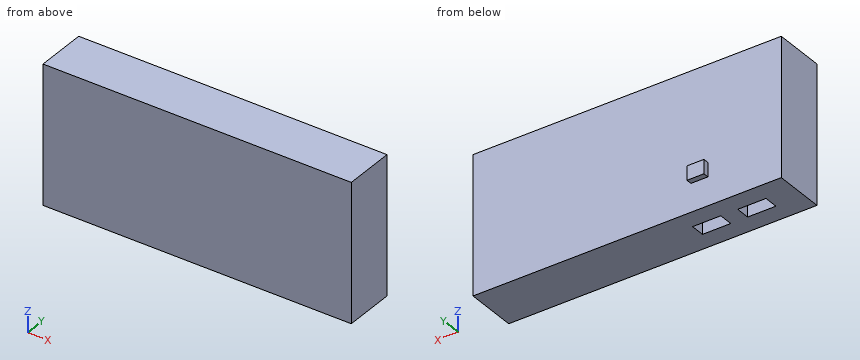
from build123d import *

# Parameters (mm, degrees)
SKETCH1_W           = 138.684
SKETCH1_H           = 62.1284
BOSS_EXTRUDE1_DEPTH = 11.43
SKETCH3_W           = 12.7
SKETCH3_H           = 6.35
CUT_EXTRUDE1_DEPTH  = 12.7
SKETCH4_W           = 7.62
SKETCH4_H           = 6.35
BOSS_EXTRUDE2_DEPTH = 2.54


with BuildPart() as part:
    # Sketch1 → Boss-Extrude1 (new, symmetric)
    with BuildSketch(Plane(origin=(0, 0, 0), x_dir=(1, 0, 0), z_dir=(0, 1, 0))):
        Rectangle(SKETCH1_W, SKETCH1_H)
    extrude(amount=BOSS_EXTRUDE1_DEPTH, both=True)

    # Sketch3 → Cut-Extrude1 (cut)
    with BuildSketch(Plane(origin=(0, 0, -31.0642), x_dir=(-1, 0, 0), z_dir=(0, 0, -1))):
        with Locations((29.972, 0)):
            Rectangle(SKETCH3_W, SKETCH3_H)
        with Locations((50.292, 0)):
            Rectangle(SKETCH3_W, SKETCH3_H)
    extrude(amount=-CUT_EXTRUDE1_DEPTH, mode=Mode.SUBTRACT)

    # Sketch4 → Boss-Extrude2 (add)
    with BuildSketch(Plane(origin=(0, 11.43, 0), x_dir=(1, 0, 0), z_dir=(0, 1, 0))):
        with Locations((-32.512, 15.1892)):
            Rectangle(SKETCH4_W, SKETCH4_H)
    extrude(amount=BOSS_EXTRUDE2_DEPTH)


solid = part.part
Geometry: final body of the model. Coordinates: model frame, mm. Give positions to 0.01 mm unless a question says otherwise; leave off trailing zeros. Write each loop counter-clockwise with the first axis right and the second up, starting at its lowest first coordinate (ties: lowest second). Pieces come first, ordered by that corner, then holes. Notation, with made-up numbers: M 54,17.5 L 109,17.5 A20 cw 109,32.5 Z; hole C 36.25,-35.75 d8. An arc over 180 degrees is marked long. Answer in a Markdown table with one row per item. Add a question column.
(1) Section A-A on z = -25.5. Return loops of the section in (x, y) (3 decimals).
(2) Section B-B on x = -30. Return loops of the section in (y, z) (3 decimals), and give its area (3 significant figures).
(3) Section D-D on z = -8. Return loops of the section in (x, y).
(4) Section C-C on y = -0.5. Return loops of the section in (x, z), and give its area (3 significant figures).
(5) Ray query, line 1 (X direction, y = -1.25, z = -22); line 2 (Z direction, x = -54.5, y = 1.25); line 3 (Z direction, x = -33.5, y = 11.5). Return the intervals inside material, ascending.
(6) First-contact query: pin 1 (14 mm diameter, centred on x = -51, z = -22, fed in from +Y); pin 2 (18.5 mm diameter, centred on x = -24, z = -12.5, fed in from +Y); pin 3 (1.3 mm diameter, centred on x = -31, y = 13, fed in from +Z); pin 4 (1.9 mm diameter, centred on x = -47, y = -1, fed in from -Z). Flat tips, straight axial feed; report the tip coordinate or a pass-through.
Result set:
| question | item | result |
|---|---|---|
| 1 | outline | M -69.342,-11.43 L 69.342,-11.43 L 69.342,11.43 L -69.342,11.43 Z; hole M -56.642,-3.175 L -43.942,-3.175 L -43.942,3.175 L -56.642,3.175 Z; hole M -36.322,-3.175 L -23.622,-3.175 L -23.622,3.175 L -36.322,3.175 Z |
| 2 | outline | M -11.43,-31.064 L -3.175,-31.064 L -3.175,-18.364 L 3.175,-18.364 L 3.175,-31.064 L 11.43,-31.064 L 11.43,-18.364 L 13.97,-18.364 L 13.97,-12.014 L 11.43,-12.014 L 11.43,31.064 L -11.43,31.064 Z |
| 2 | area | 1,360 mm^2 |
| 3 | outline | M -69.34,-11.43 L 69.34,-11.43 L 69.34,11.43 L -69.34,11.43 Z |
| 4 | outline | M -69.34,-31.06 L -56.64,-31.06 L -56.64,-18.36 L -43.94,-18.36 L -43.94,-31.06 L -36.32,-31.06 L -36.32,-18.36 L -23.62,-18.36 L -23.62,-31.06 L 69.34,-31.06 L 69.34,31.06 L -69.34,31.06 Z |
| 4 | area | 8,290 mm^2 |
| 5 | line 1 | x = -69.34 to -56.64, -43.94 to -36.32, -23.62 to 69.34 |
| 5 | line 2 | z = -18.36 to 31.06 |
| 5 | line 3 | z = -18.36 to -12.01 |
| 6 | pin 1 | stops at y = 11.43 |
| 6 | pin 2 | stops at y = 13.97 |
| 6 | pin 3 | stops at z = -12.01 |
| 6 | pin 4 | stops at z = -18.36 |
